```python
from build123d import *

# Parameters (mm, degrees)
F0_R     = 10.9982
F1_DEPTH = 7.9756
F3_DEPTH = 7.9756
F4_W     = 4.070462
F4_H     = 10.939364
F5_DEPTH = 7.9756
F6_R     = 1.5875


with BuildPart() as f1:
    # F0 (on Top) → F1 (new body)
    with BuildSketch(Plane.XY):
        with BuildLine():
            ThreePointArc((11.950254, 20.352071), (0, 21.486685), (-11.950254, 20.352071))
            Line((-11.950254, 20.352071), (-16.087743, 19.559259))
            ThreePointArc((-16.087743, 19.559259), (-19.787148, 17.368341), (-21.242717, 13.32272))
            Line((-21.242717, 13.32272), (-21.242717, 0))
            Line((-21.242717, 0), (-21.242717, -13.32272))
            ThreePointArc((-21.242717, -13.32272), (-19.787148, -17.368341), (-16.087743, -19.559259))
            Line((-16.087743, -19.559259), (-11.950254, -20.352071))
            ThreePointArc((-11.950254, -20.352071), (0, -21.486685), (11.950254, -20.352071))
            Line((11.950254, -20.352071), (16.087743, -19.559259))
            ThreePointArc((16.087743, -19.559259), (19.787148, -17.368341), (21.242717, -13.32272))
            Line((21.242717, -13.32272), (21.242717, 0))
            Line((21.242717, 0), (21.242717, 13.32272))
            ThreePointArc((21.242717, 13.32272), (19.787148, 17.368341), (16.087743, 19.559259))
            Line((16.087743, 19.559259), (11.950254, 20.352071))
        make_face()
        Circle(F0_R, mode=Mode.SUBTRACT)
    extrude(amount=F1_DEPTH)



with BuildPart() as f3:
    # F2 (on Top) → F3 (new body)
    with BuildSketch(Plane.XY):
        with BuildLine():
            ThreePointArc((-22.1818, 35.461367), (-33.585531, 28.984005), (-38.1, 16.670563))
            Line((-38.1, 16.670563), (-38.1, -16.670563))
            ThreePointArc((-38.1, -16.670563), (-33.585531, -28.984005), (-22.1818, -35.461367))
            Line((-22.1818, -35.461367), (-6.35, -38.1))
            Line((-6.35, -38.1), (-6.35, -25.224819))
            Line((-6.35, -25.224819), (-20.093933, -22.934164))
            ThreePointArc((-20.093933, -22.934164), (-23.895177, -20.775043), (-25.4, -16.670563))
            Line((-25.4, -16.670563), (-25.4, 16.670563))
            ThreePointArc((-25.4, 16.670563), (-23.895177, 20.775043), (-20.093933, 22.934164))
            Line((-20.093933, 22.934164), (-6.35, 25.224819))
            Line((-6.35, 25.224819), (-6.35, 38.1))
            Line((-6.35, 38.1), (-22.1818, 35.461367))
        make_face()
        with BuildLine():
            Line((38.1, -16.670563), (38.1, 16.670563))
            ThreePointArc((38.1, 16.670563), (33.585531, 28.984005), (22.1818, 35.461367))
            Line((22.1818, 35.461367), (6.35, 38.1))
            Line((6.35, 38.1), (6.35, 25.224819))
            Line((6.35, 25.224819), (20.093933, 22.934164))
            ThreePointArc((20.093933, 22.934164), (23.895177, 20.775043), (25.4, 16.670563))
            Line((25.4, 16.670563), (25.4, -16.670563))
            ThreePointArc((25.4, -16.670563), (23.895177, -20.775043), (20.093933, -22.934164))
            Line((20.093933, -22.934164), (6.35, -25.224819))
            Line((6.35, -25.224819), (6.35, -38.1))
            Line((6.35, -38.1), (22.1818, -35.461367))
            ThreePointArc((22.1818, -35.461367), (33.585531, -28.984005), (38.1, -16.670563))
        make_face()
    extrude(amount=F3_DEPTH)


with BuildPart() as f1_1:
    add(f1.part)

    add(f3.part)  # F5 merges F3
    # F4 (on Top) → F5 (join)
    with BuildSketch(Plane.XY):
        with Locations((-13.865008, 21.497123)):
            Rectangle(F4_W, F4_H)
        with Locations((13.865008, 21.497123)):
            Rectangle(F4_W, F4_H)
        with Locations((13.865008, -21.497123)):
            Rectangle(F4_W, F4_H)
        with Locations((-13.865008, -21.497123)):
            Rectangle(F4_W, F4_H)
    extrude(amount=F5_DEPTH)

    # F6
    f6_edges = [f1_1.edges().sort_by_distance(p)[0] for p in [
        (-14.2659, -36.780683, 7.9756),
        (14.2659, -36.780683, 7.9756),
        (14.2659, -36.780683, 0),
        (-14.2659, -36.780683, 0),
    ]]
    fillet(f6_edges, radius=F6_R)


solid = f1_1.part
```
Geometry check sheet. Reference: the model listing, model coordinates, mm. A direction names the side the tool comes from. Coordinates: 2 decimals unless noted, no trailing zeros. Order: outer loops, then holes, each group sorted by start corner. A loop starts at its lowest first (then second) coordinate and runs counter-clockwise, first axis right, second up. Notation, with made-up numbers: M 56,81.5 L 69,81.5 A10 ccw 69,86.5 Z; hole C -34.75,-28 d11. An arc over 180 degrees is marked long. One line per question, with ' | ' between items. Start each with the question number.
Item 1: Material ranges on L1, parallel to X at y = 12, z = 5; L2, parallel to Y at x = 0, z = 5.75; L3, parallel to Y at x = -20.5, z = 2.75, recorded low to high. Write a range as [from, to].
Item 2: Cross-section at C-C on z = 3. State how many separate pieces and enclosed holes the cut face has, then the cut area to 3 significant figures.
Item 3: Cross-section at A-A on x = 0. Enter the section's corners in (y, z).
Item 4: Cross-section at B-B on y = 0. Enter the section's corners in (x, z) (1 decimal).
Item 5: Draft check along Y on faces 4 (the flat face through (-11.83, -22, 4)), 5 (the flat face through (38.1, 0, 4)), 6 (the flat face through (-14.16, 36.8, 3.95)), 7 (the cylindrical face through (-0.167, -21.486, 3.932)). Enter one of: pulls with the +Y half, pulls with the -Y half, needs draft (parallel to the pull), parting line crosses it, or undercut.
Item 6: Gauge pin test, flat ends, axial feed: pin 1 (5 mm diameter, centred on x = -9.5, y = -2.5, fed in from +Z); pin 2 (4.5 mm diameter, centred on y = -21.5, z = 5, fed in from -X); pin 3 (13 mm diameter, centred on x = 0, y = 0, fed in from +Z); pin 4 (4.5 mm diameter, centred on y = -22.5, z = 4, fed in from -X). Record the tip position at first contact, or that the pin passes through.
Item 7: Set-up check for faces 1 (the flat face through (6.35, -32, 4)), 2 (the cylindrical face through (-33.46, 29.13, 3.95)), 3 (the flat face through (11.83, -22, 4)): record each of +Z, -Z, +X, -X, +Y, -Y from which the full face is reachable in a straight line by a thin tool's end or side.
Findings:
1) L1: x = [-38.1, -25.4], [-21.24, 21.24], [25.4, 38.1] | L2: y = [-21.49, -11], [11, 21.49] | L3: y = [-35.74, -22.85], [-16.3, 16.3], [22.85, 35.74]
2) separate pieces: 1 | enclosed holes: 3 | area: 3,910 mm²
3) outline: M -21.49,0 L -11,0 L -11,7.98 L -21.49,7.98 Z; M 11,0 L 21.49,0 L 21.49,7.98 L 11,7.98 Z
4) outline: M -38.1,1.6 A1.6 ccw -36.5,0 L -25.4,0 L -25.4,8 L -36.5,8 A1.6 ccw -38.1,6.4 Z; M -21.2,0 L -11,0 L -11,8 L -21.2,8 Z; M 11,0 L 21.2,0 L 21.2,8 L 11,8 Z; M 25.4,0 L 36.5,0 A1.6 ccw 38.1,1.6 L 38.1,6.4 A1.6 ccw 36.5,8 L 25.4,8 Z
5) face 4: undercut | face 5: needs draft | face 6: pulls with the +Y half | face 7: undercut
6) pin 1: stops at z = 7.98 | pin 2: stops at x = -37.92 | pin 3: passes through | pin 4: stops at x = -37.76
7) face 1: +Z, -Z, -Y | face 2: +Z, -Z, -X, +Y | face 3: +Z, -Z
